Geometry check sheet. Reference: the model listing, model coordinates, mm. A direction names the side the tool comes from. Round coordinates to 2 decimals unless told otherwise and drop trailing zeros. Order: outer loops, then holes, each group sorted by start corner. A loop starts at its lowest first (then second) coordinate and runs counter-clockwise, first axis right, second up. Notation, with made-up numbers: (10.5, 81) -> (27.5, 81) arc R19 cw to (27.5, 90) -> close; hole circle Ø7 at (67.25, -29). An arc over 180 degrees is marked (long way). Use a Markdown table: item, result. Add a question column.
Item 1: Sectioned sample at A-A, the plane z = 2.25. Record the cut outline in (x, y).
Item 2: Gauge pin test, flat ends, axial feed: pin 1 Ø1 at (x, z) = (11, 2.5) entering from +Y; pin 2 Ø6 at (x, y) = (5.3, 5.3) entering from +Z; pin 3 Ø3 at (x, z) = (5, 1) entering from +Y. Record the tip position at first contact, or that the pin passes through.
Item 3: Set-up check for faces 1 (the flat face through (0, 3, 0)), 2 (the cylindrical face through (4.219, 0.422, 4.254)), 3 (the cylindrical face through (-0.59, 4.46, 1.48)): record each of +Z, -Z, +X, -X, +Y, -Y from which the full face is reachable in a straight line by a thin tool's end or side.
Item 4: Material ranges on probe 1 along Y at (x, z) = (0, 2); probe 2 along X at (y, z) = (-4, 0.9); probe 3 along Y at (x, z) = (-2.5, 2.9), recorded low to high. Write a range as [from, to].
Item 5: Mould release check, pull along X, two halves, no side actions. Record for faces 4 (the cylindrical face through (-14.985, -0.66, 2.028)), 5 (the flat face through (-0.1, -13.4, 0)), 6 (the flat face through (6, 0, 3)): pulls with the +X half, pulls with the -X half, needs draft (parallel to the pull), parting line crosses it, or undercut.
from build123d import *

# Parameters (mm, degrees)
SKETCH_R      = 4.5
PAD_DEPTH     = 3
SKETCH001_R   = 15
PAD001_DEPTH  = 2
SKETCH002_R   = 15
SKETCH002_R_2 = 13
PAD002_DEPTH  = 3
SKETCH003_R   = 5
POCKET_DEPTH  = 1
FILLET_R      = 0.5
CHAMFER_SIZE  = 1


with BuildPart() as part:
    # Sketch → Pad (new body)
    with BuildSketch(Plane.XY):
        Circle(SKETCH_R)
        with BuildLine():
            ThreePointArc((-2.059126, 2.25), (0, -3.05), (2.059126, 2.25))
            Line((-2.059126, 2.25), (2.059126, 2.25))
        make_face(mode=Mode.SUBTRACT)
    extrude(amount=PAD_DEPTH)

    # Sketch001 (on Face5 of Pad) → Pad001 (join)
    with BuildSketch(Plane.XY.offset(3)):
        Circle(SKETCH001_R)
    extrude(amount=PAD001_DEPTH)

    # Sketch002 (on Face2 of Pad001) → Pad002 (join)
    with BuildSketch(Plane(origin=(0, 0, 3), x_dir=(1, 0, 0), z_dir=(0, 0, -1))):
        Circle(SKETCH002_R)
        Circle(SKETCH002_R_2, mode=Mode.SUBTRACT)
    extrude(amount=PAD002_DEPTH)

    # Sketch003 (on Face3 of Pad002) → Pocket (cut)
    with BuildSketch(Plane.XY.offset(5)):
        with Locations((5.303301, 5.303301)):
            Circle(SKETCH003_R)
    extrude(amount=-POCKET_DEPTH, mode=Mode.SUBTRACT)

    # Fillet
    fillet_edges = [part.edges().sort_by_distance(p)[0] for p in [
        (0.303301, 5.303301, 5),
    ]]
    fillet(fillet_edges, radius=FILLET_R)

    # Chamfer
    chamfer_edges = [part.edges().sort_by_distance(p)[0] for p in [
        (-15, 0, 5),
    ]]
    chamfer(chamfer_edges, length=CHAMFER_SIZE)


solid = part.part
Found:
| question | item | result |
|---|---|---|
| 1 | outline | circle Ø30 at (0, 0); circle Ø9 at (0, 0); hole circle Ø26 at (0, 0); hole (-2.06, 2.25) arc R3.05 ccw (long way) to (2.06, 2.25) -> close |
| 2 | pin 1 | stops at y = 10.71 |
| 2 | pin 2 | stops at z = 4 |
| 2 | pin 3 | stops at y = 14.59 |
| 3 | face 1 | -Z, +X, -X, +Y, -Y |
| 3 | face 2 | +Z |
| 3 | face 3 | -Z |
| 4 | probe 1 | y = [-15, -13], [-4.5, -3.05], [2.25, 4.5], [13, 15] |
| 4 | probe 2 | x = [-14.46, -12.37], [-2.06, 2.06], [12.37, 14.46] |
| 4 | probe 3 | y = [-14.79, -12.76], [-3.74, -1.75], [1.75, 3.74], [12.76, 14.79] |
| 5 | face 4 | parting line crosses it |
| 5 | face 5 | needs draft |
| 5 | face 6 | undercut |
